from build123d import *

# Parameters (mm, degrees)
F0_W      = 29
F0_H      = 16.5
F1_DEPTH  = 38.5
F2_T      = -2
F3_DEPTH  = 2.25
F4_SIZE   = 2
F5_SIZE   = 2
F6_SIZE   = 1
F8_DEPTH  = 16.501
F9_W      = 12.5
F9_H      = 1
F10_DEPTH = 2
F11_R     = 2
F12_DEPTH = 2.001
F13_W     = 7.54
F13_H     = 7.25
F13_R     = 1.1
F14_DEPTH = 4.35
F17_W     = 5.538
F17_H     = 4.583
F15_W     = 5.538
F15_H     = 5.533


with BuildPart() as f1:
    # F0 (on Top) → F1 (new body)
    with BuildSketch(Plane.XY):
        with Locations((14.5, 8.25)):
            Rectangle(F0_W, F0_H)
    extrude(amount=F1_DEPTH)

    # F2
    f2_openings = [f1.faces().sort_by_distance(p)[0] for p in [
        (14.5, 8.25, 38.5),
    ]]
    offset(amount=F2_T, openings=f2_openings)

    # F3 (add): a face of the model
    f3_faces = [f1.faces().sort_by_distance(p)[0] for p in [
        (14.5, 8.25, 2),
    ]]
    extrude(f3_faces, amount=F3_DEPTH)

    # F4
    f4_edges = [f1.edges().sort_by_distance(p)[0] for p in [
        (29, 0, 19.25),
        (0, 0, 19.25),
        (29, 16.5, 19.25),
        (0, 16.5, 19.25),
    ]]
    chamfer(f4_edges, length=F4_SIZE)

    # F5
    f5_edges = [f1.edges().sort_by_distance(p)[0] for p in [
        (0, 8.25, 0),
        (1, 15.5, 0),
        (1, 1, 0),
        (14.5, 16.5, 0),
        (14.5, 0, 0),
        (28, 15.5, 0),
        (28, 1, 0),
        (29, 8.25, 0),
    ]]
    chamfer(f5_edges, length=F5_SIZE)

    # F6
    f6_edges = [f1.edges().sort_by_distance(p)[0] for p in [
        (14.5, 0, 38.5),
        (1, 1, 38.5),
        (0, 8.25, 38.5),
        (1, 15.5, 38.5),
        (14.5, 16.5, 38.5),
        (28, 15.5, 38.5),
        (29, 8.25, 38.5),
        (28, 1, 38.5),
    ]]
    chamfer(f6_edges, length=F6_SIZE)

    # F7 (on face) → F8 (cut, through all)
    with BuildSketch(Plane.XZ):
        Polygon((6.464, 8.664), (6.464, 4.94), (23.536, 4.94), (23.536, 8.664), (17.364, 12.834), (12.635, 12.834), align=None)
    extrude(amount=-F8_DEPTH, mode=Mode.SUBTRACT)

    # F9 (on face) → F10 (cut, through all)
    with BuildSketch(Plane.YZ.offset(29)):
        with BuildLine():
            ThreePointArc((5.0038961688, 23.1590909091), (8.25, 22.25), (11.4961038312, 23.1590909091))
            ThreePointArc((11.4961038312, 23.1590909091), (8.25, 26.25), (5.0038961688, 23.1590909091))
        make_face()
        with BuildLine():
            ThreePointArc((5.0038961688, 23.1590909091), (8.1704306945, 19.7509741882), (11.5, 23))
            ThreePointArc((11.5, 23), (11.4990258118, 23.0795693055), (11.4961038312, 23.1590909091))
            ThreePointArc((11.4961038312, 23.1590909091), (8.25, 22.25), (5.0038961688, 23.1590909091))
        make_face()
        with BuildLine():
            ThreePointArc((5.0038961688, 23.1590909091), (8.25, 26.25), (11.4961038312, 23.1590909091))
            ThreePointArc((11.4961038312, 23.1590909091), (13.6975062618, 25.4361502113), (14.5, 28.5))
            Line((14.5, 28.5), (2, 28.5))
            ThreePointArc((2, 28.5), (2.8024937382, 25.4361502113), (5.0038961688, 23.1590909091))
        make_face()
        with BuildLine():
            Line((2, 28.5), (14.5, 28.5))
            ThreePointArc((14.5, 28.5), (8.25, 34.75), (2, 28.5))
        make_face()
        with BuildLine():
            ThreePointArc((2, 28.5), (8.25, 34.75), (14.5, 28.5))
            Line((14.5, 28.5), (14.5, 37.5))
            Line((14.5, 37.5), (2, 37.5))
            Line((2, 37.5), (2, 28.5))
        make_face()
        with Locations((8.25, 38)):
            Rectangle(F9_W, F9_H)
    extrude(amount=-F10_DEPTH, mode=Mode.SUBTRACT)

    # F11 (on face) → F12 (cut, through all)
    with BuildSketch(Plane.YZ.offset(2)):
        with Locations((8.25, 23)):
            Circle(F11_R)
    extrude(amount=-F12_DEPTH, mode=Mode.SUBTRACT)

    # F13 (on face) → F14 (join)
    with BuildSketch(Plane(origin=(27, 0, 0), x_dir=(0, -1, 0), z_dir=(-1, 0, 0))):
        with Locations((-8.25, 7.875)):
            Rectangle(F13_W, F13_H)
        with Locations((-8.25, 9)):
            Circle(F13_R, mode=Mode.SUBTRACT)
    extrude(amount=F14_DEPTH)

    # F17 (on offset) → F18 section 0
    with BuildSketch(Plane.YZ.offset(24.55)):
        with Locations((8.25, 8.5135)):
            Rectangle(F17_W, F17_H)
    # F15 (on face) → F18 section 1
    with BuildSketch(Plane.YZ.offset(29)):
        with Locations((8.25, 8.0385)):
            Rectangle(F15_W, F15_H)
    loft(mode=Mode.SUBTRACT)


solid = f1.part
Geometry: final body of the model. Coordinates: model frame, mm. A direction names the side the tool comes from. Give positions to 0.01 mm unless a question says otherwise; leave off trailing zeros. Write each loop counter-clockwise with the first axis right and the second up, starting at its lowest first coordinate (ties: lowest second). Pieces come first, ordered by that corner, then holes. Notation, with made-up numbers: (86, 26) -> (115, 26) arc R32 cw to (115, 64) -> close; hole circle Ø7 at (50.25, 16). An arc over 180 degrees is marked (long way). Answer as a JSON object with one key per item and string values.
1. Cut plane D-D on z = 24. Output: boundary loops of the cut face in (x, y), and give its area (3 significant figures).
Ans:
{"outline": "(0, 2) -> (2, 0) -> (27, 0) -> (29, 2) -> (29, 3.91) -> (27, 3.91) -> (27, 2) -> (2, 2) -> (2, 6.52) -> (0, 6.52) -> close; (0, 9.98) -> (2, 9.98) -> (2, 14.5) -> (27, 14.5) -> (27, 12.59) -> (29, 12.59) -> (29, 14.5) -> (27, 16.5) -> (2, 16.5) -> (0, 14.5) -> close", "area": "134 mm^2"}
2. Cut plane C-C on x = 14.5. Output: boundary loops of the cut face in (y, z), and give its area (3 significant figures).
Ans:
{"outline": "(0, 2) -> (2, 0) -> (14.5, 0) -> (16.5, 2) -> (16.5, 4.94) -> (14.5, 4.94) -> (14.5, 4.25) -> (2, 4.25) -> (2, 4.94) -> (0, 4.94) -> close; (0, 12.83) -> (2, 12.83) -> (2, 38.5) -> (1, 38.5) -> (0, 37.5) -> close; (14.5, 12.83) -> (16.5, 12.83) -> (16.5, 37.5) -> (15.5, 38.5) -> (14.5, 38.5) -> close", "area": "171 mm^2"}
3. Mould query, pull axis X, two halves, no side actions, for faces 1 (the flat face through (28, 1, 20)), 2 (the flat face through (14, 1, 1)), 3 (the flat face through (23.536, 15, 7)). Classes: pulls with the +X half, pulls with the -X half, needs draft (parallel to the pull), parting line crosses it, or undercut.
Ans:
{"face 1": "pulls with the +X half", "face 2": "needs draft", "face 3": "undercut"}
4. Cut plane B-B on z = 18. Output: boundary loops of the cut face in (x, y), and give its area (3 significant figures).
Ans:
{"outline": "(0, 2) -> (2, 0) -> (27, 0) -> (29, 2) -> (29, 14.5) -> (27, 16.5) -> (2, 16.5) -> (0, 14.5) -> close; hole (2, 2) -> (27, 2) -> (27, 14.5) -> (2, 14.5) -> close", "area": "158 mm^2"}
5. Ray query, probe 1 along Y at (x, z) = (25, 6); probe 2 along Y at (x, z) = (23.7, 9); probe 3 along X at (y, z) = (12, 23). Return the intervals inside material, ascending. Write a range as from..to.
Ans:
{"probe 1": "y = 0..2, 4.48..12.02, 14.5..16.5", "probe 2": "y = 0..2, 4.48..7.15, 9.35..12.02, 14.5..16.5", "probe 3": "x = 0..2, 27..29"}
6. Access query for faces 4 (the cylindrical face through (23.613, 7.234, 8.579)), 5 (the flat face through (23.536, 1, 7)), 6 (the flat face through (6.464, 15, 7)), 7 (the flat face through (15, 2, 25)). Directions: +Z, -Z, +X, -X, +Y, -Y. A direction counts if a zero-diameter tool reaches every point of the face in a straight line with its end or side. Return the directions, or none.
Ans:
{"face 4": "+X", "face 5": "-Y", "face 6": "+Y, -Y", "face 7": "+Z"}
7. Contact query for flat-ended pins moving along their axis: pin 1 (1.5 mm diameter, centred on x = 21.5, y = 12, fed in from +Z); pin 2 (0.6 mm diameter, centred on y = 1, z = 7, fed in from +X); pin 3 (3.5 mm diameter, centred on x = 25.5, y = 7, fed in from +Z). Output: stop coordinate, or through.
Ans:
{"pin 1": "stops at z = 4.25", "pin 2": "stops at x = 28.3", "pin 3": "stops at z = 20.56"}
8. Cut plane A-A on y = 8.25. Output: boundary loops of the cut face in (x, z) (3 decimals), and give its area (3 significant figures).
Ans:
{"outline": "(0, 2) -> (2, 0) -> (27, 0) -> (29, 2) -> (29, 5.272) -> (24.55, 6.222) -> (24.55, 7.9) -> (22.65, 7.9) -> (22.65, 4.25) -> (2, 4.25) -> (2, 21) -> (0, 21) -> close; (0, 25) -> (2, 25) -> (2, 38.5) -> (1, 38.5) -> (0, 37.5) -> close; (22.65, 10.1) -> (24.55, 10.1) -> (24.55, 10.805) -> (29, 10.805) -> (29, 19.75) -> (27, 19.75) -> (27, 11.5) -> (22.65, 11.5) -> close", "area": "215 mm^2"}
